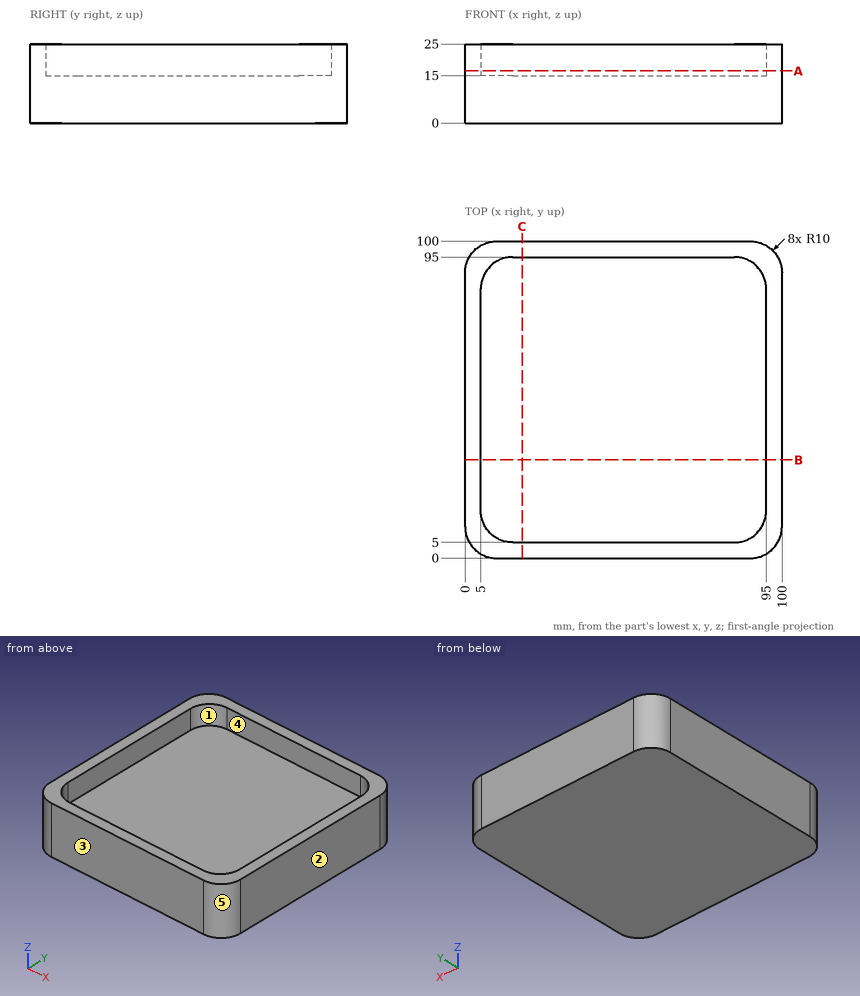
The figure shows three views and two pictorial views of one solid part (mm, origin at its lowest corner). Answer the questions. A direction names the side the tool comes from. Coordinates: 2 decimals unless noted, no trailing zeros. Write each loop counter-clockwise with the first axis right and the second up, starting at its lowest first coordinate (ties: lowest second). Pieces come first, ordered by that corner, then holes. Notation, with made-up numbers: (34, 48) -> (67, 48) arc R33 ccw to (67, 83) -> close; hole circle Ø7 at (23.25, -40). An arc over 180 degrees is marked (long way). Return JSON: item names as keys, results as strings.
(1) Consider line 1 along X through (y, z) = (34.5, 18.5); line 2 along Y through (x, z) = (9.5, 14). Determine where each line is inside the solid, lowest interval first. Write a range as from..to.
Answers below:
{"line 1": "0..5, 95..100", "line 2": "0.01..99.99"}
(2) The part is cut by section B-B on y = 31. Give the vertices of the cut face in (x, z).
Answers below:
{"outline": "(0, 0) -> (100, 0) -> (100, 25) -> (95, 25) -> (95, 15) -> (5, 15) -> (5, 25) -> (0, 25) -> close"}
(3) Which of the six approach directions +Z, -Z, +X, -X, +Y, -Y give full straight-line access (tool end or side, diameter ignored) to the marked faces 4 and 5?
Answers below:
{"face 4": "+Z", "face 5": "+Z, -Z, +X, -Y"}
(4) For a pull along Y with two mould halves and no side action, classify the marked faces 1, 2 and 3 as pulls with the +Y half, pulls with the -Y half, needs draft (parallel to the pull), parting line crosses it, or undercut.
Answers below:
{"face 1": "undercut", "face 2": "needs draft", "face 3": "pulls with the -Y half"}
(5) Each of these flat-tipped pins is pushed along its axis until it touches: P1, Ø1, axis at x = 44, y = 66, coming from the -Z side; P2, Ø5, axis at x = 27, y = 20, coming from the +Z side. Where does it stop, or does it pass through?
Answers below:
{"P1": "z = 0", "P2": "z = 15"}
(6) The part is cut by section A-A on z = 16.5. Give the vertices of the cut face in (x, y), then the cut area to 3 significant figures.
Answers below:
{"outline": "(0, 10) arc R10 ccw to (10, 0) -> (90, 0) arc R10 ccw to (100, 10) -> (100, 90) arc R10 ccw to (90, 100) -> (10, 100) arc R10 ccw to (0, 90) -> close; hole (5, 15) arc R10 ccw to (15, 5) -> (85, 5) arc R10 ccw to (95, 15) -> (95, 85) arc R10 ccw to (85, 95) -> (15, 95) arc R10 ccw to (5, 85) -> close", "area": "1,900 mm^2"}
